Answer from the drawing. Dimensions are ordinates in mm from the lowest x, y and z of the part. A direction names the side the tool comes from. Round coordinates to 2 decimals unless told otherwise and drop trailing zeros. Write each loop counter-clockwise with the first axis right and the second up, starting at its lowest first coordinate (ties: lowest second). Pieces come first, ordered by that corner, then holes. Notation, with made-up numbers: (-20.5, -26) - (-6.5, -26) arc R22 cw to (-6.5, -8) - close; hole circle Ø3 at (45, 36). An arc over 180 degrees is marked (long way). Answer in a Markdown table with one row per item.
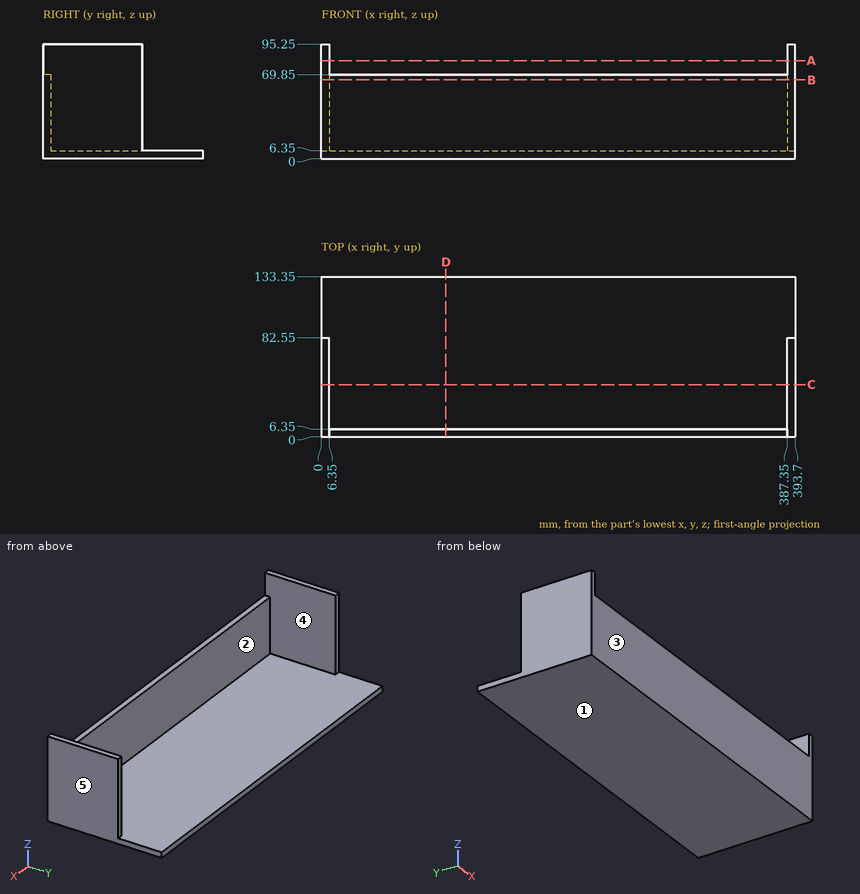
(1) Flat-ended cylindrical pins translate along their axes: pin 1 (3 mm diameter, centred on x = 166.5, z = 51.5, fed in from +Y); pin 2 (1 mm diameter, centred on x = 118.5, y = 86, fed in from +Z); pin 3 (5 mm diameter, centred on x = 2.5, z = 45, fed in from +Y). Find the tip coordinate at first contact, or state that the pin passes through.
Checked values:
| item | result |
|---|---|
| pin 1 | stops at y = 6.35 |
| pin 2 | stops at z = 6.35 |
| pin 3 | stops at y = 82.55 |
(2) Section A-A (z = 81.5) is taken. Give the vertices of the cut face in (x, y).
Checked values:
| item | result |
|---|---|
| outline | (0, 0) - (6.35, 0) - (6.35, 82.55) - (0, 82.55) - close; (387.35, 0) - (393.7, 0) - (393.7, 82.55) - (387.35, 82.55) - close |
(3) Section D-D (x = 103.5) is taken. Give the vertices of the cut face in (y, z).
Checked values:
| item | result |
|---|---|
| outline | (0, 0) - (133.35, 0) - (133.35, 6.35) - (6.35, 6.35) - (6.35, 69.85) - (0, 69.85) - close |
(4) For the marked faces 1 and 2, determine the directions among +Z, -Z, +X, -X, +Y, -Y from which every point of the face is accessible in a straight line to the end or side of a thin tool.
Checked values:
| item | result |
|---|---|
| face 1 | -Z, +X, -X, +Y, -Y |
| face 2 | +Z, +Y |
(5) For a pull along X with two mould halves and no side action, classify the marked faces 3, 4 and 5 as pulls with the +X half, pulls with the -X half, needs draft (parallel to the pull), parting line crosses it, or undercut.
Checked values:
| item | result |
|---|---|
| face 3 | needs draft |
| face 4 | undercut |
| face 5 | pulls with the +X half |
(6) Find the intervals of material crossed by line 1 (X direction, y = 64, z = 15.5); line 2 (Y direction, x = 369.5, z = 20), in increasing order.
Checked values:
| item | result |
|---|---|
| line 1 | x = 0 to 6.35, 387.35 to 393.7 |
| line 2 | y = 0 to 6.35 |
(7) Section C-C (y = 43.5) is taken. Give the vertices of the cut face in (x, z), and give its area (3 significant figures).
Checked values:
| item | result |
|---|---|
| outline | (0, 0) - (393.7, 0) - (393.7, 95.25) - (387.35, 95.25) - (387.35, 6.35) - (6.35, 6.35) - (6.35, 95.25) - (0, 95.25) - close |
| area | 3,630 mm2 |
(8) Section B-B (z = 65.5) is taken. Give the vertices of the cut face in (x, y).
Checked values:
| item | result |
|---|---|
| outline | (0, 0) - (393.7, 0) - (393.7, 82.55) - (387.35, 82.55) - (387.35, 6.35) - (6.35, 6.35) - (6.35, 82.55) - (0, 82.55) - close |
